from build123d import *

# Parameters (mm, degrees)
ESBO_O1_R                = 2.4
ESBO_O1_W                = 30
ESBO_O1_H                = 4
RESSALTO_EXTRUS_O1_DEPTH = 4
ESBO_O3_R                = 4
CORTE_EXTRUS_O1_DEPTH    = 6
FURO_COM_FOLGA_DE_M41_D  = 4.5
RESSALTO_EXTRUS_O2_DEPTH = 4
ESBO_O8_R                = 6
ESBO_O8_R_2              = 9
CORTE_EXTRUS_O4_DEPTH    = 5


with BuildPart() as part:
    # Esboço1 → Ressalto-extrusão1 (new body)
    with BuildSketch(Plane.XY):
        with BuildLine():
            Line((120, 130), (120, 140))
            ThreePointArc((120, 140), (122.928932188, 147.071067812), (130, 150))
            Line((130, 150), (50, 150))
            ThreePointArc((50, 150), (57.071067812, 147.071067812), (60, 140))
            Line((60, 140), (60, 130))
            Line((60, 130), (120, 130))
        make_face()
        with BuildLine():
            Line((0, 140), (0, 0))
            Line((0, 0), (400, 0))
            Line((400, 0), (400, 140))
            ThreePointArc((400, 140), (397.071067812, 147.071067812), (390, 150))
            Line((390, 150), (319, 150))
            Line((319, 150), (301, 150))
            Line((301, 150), (130, 150))
            ThreePointArc((130, 150), (122.928932188, 147.071067812), (120, 140))
            Line((120, 140), (120, 130))
            Line((120, 130), (60, 130))
            Line((60, 130), (60, 140))
            ThreePointArc((60, 140), (57.071067812, 147.071067812), (50, 150))
            Line((50, 150), (10, 150))
            ThreePointArc((10, 150), (2.928932188, 147.071067812), (0, 140))
        make_face()
        with Locations((30, 96.5)):
            Circle(ESBO_O1_R, mode=Mode.SUBTRACT)
        with Locations((30, 133.5)):
            Circle(ESBO_O1_R, mode=Mode.SUBTRACT)
        with Locations((100, 126)):
            Rectangle(ESBO_O1_W, ESBO_O1_H, mode=Mode.SUBTRACT)
        with BuildLine():
            ThreePointArc((365, 94.1), (362.6, 96.5), (365, 98.9))
            Line((365, 98.9), (375, 98.9))
            ThreePointArc((375, 98.9), (377.4, 96.5), (375, 94.1))
            Line((375, 94.1), (365, 94.1))
        make_face(mode=Mode.SUBTRACT)
        with Locations((200, 126)):
            Rectangle(ESBO_O1_W, ESBO_O1_H, mode=Mode.SUBTRACT)
        with Locations((300, 126)):
            Rectangle(ESBO_O1_W, ESBO_O1_H, mode=Mode.SUBTRACT)
        with BuildLine():
            ThreePointArc((365, 131.1), (362.6, 133.5), (365, 135.9))
            Line((365, 135.9), (375, 135.9))
            ThreePointArc((375, 135.9), (377.4, 133.5), (375, 131.1))
            Line((375, 131.1), (365, 131.1))
        make_face(mode=Mode.SUBTRACT)
    extrude(amount=RESSALTO_EXTRUS_O1_DEPTH)

    # Esboço3 → Corte-extrusão1 (cut)
    with BuildSketch(Plane.XY.offset(4)):
        with Locations((30, 115)):
            Circle(ESBO_O3_R)
        with BuildLine():
            Line((365, 119), (375, 119))
            ThreePointArc((375, 119), (379, 115), (375, 111))
            Line((375, 111), (365, 111))
            ThreePointArc((365, 111), (361, 115), (365, 119))
        make_face()
        with BuildLine():
            Line((40, 67.5), (60, 67.5))
            ThreePointArc((60, 67.5), (61.5, 66), (60, 64.5))
            Line((60, 64.5), (40, 64.5))
            ThreePointArc((40, 64.5), (38.5, 66), (40, 67.5))
        make_face()
        with BuildLine():
            Line((71, 36.5), (91, 36.5))
            ThreePointArc((91, 36.5), (92.5, 35), (91, 33.5))
            Line((91, 33.5), (71, 33.5))
            ThreePointArc((71, 33.5), (69.5, 35), (71, 36.5))
        make_face()
        with BuildLine():
            Line((71, 67.5), (91, 67.5))
            ThreePointArc((91, 67.5), (92.5, 66), (91, 64.5))
            Line((91, 64.5), (71, 64.5))
            ThreePointArc((71, 64.5), (69.5, 66), (71, 67.5))
        make_face()
        with BuildLine():
            Line((40, 36.5), (60, 36.5))
            ThreePointArc((60, 36.5), (61.5, 35), (60, 33.5))
            Line((60, 33.5), (40, 33.5))
            ThreePointArc((40, 33.5), (38.5, 35), (40, 36.5))
        make_face()
        with BuildLine():
            Line((55.5, 62), (75.5, 62))
            ThreePointArc((75.5, 62), (87, 50.5), (75.5, 39))
            Line((75.5, 39), (55.5, 39))
            ThreePointArc((55.5, 39), (44, 50.5), (55.5, 62))
        make_face()
    extrude(amount=-CORTE_EXTRUS_O1_DEPTH, mode=Mode.SUBTRACT)

    # Furo com folga de M41 (through all)
    with Locations(Plane(origin=(50, 12.5, 4), x_dir=(1, 0, 0), z_dir=(0, 0, 1))):
        with Locations((0, 0), (100, 0), (200, 0), (300, 0), (225, 62.5), (75, 62.5), (27, 127.5), (80, 127.5)):
            Hole(FURO_COM_FOLGA_DE_M41_D / 2)

    # Esboço5 → Ressalto-extrusão2 (add)
    with BuildSketch(Plane.XY.offset(4)):
        with BuildLine():
            Line((0, 140), (0, 148))
            ThreePointArc((0, 148), (2.928932188, 155.071067812), (10, 158))
            Line((10, 158), (390, 158))
            ThreePointArc((390, 158), (397.071067812, 155.071067812), (400, 148))
            Line((400, 148), (400, 140))
            ThreePointArc((400, 140), (397.071067812, 147.071067812), (390, 150))
            Line((390, 150), (10, 150))
            ThreePointArc((10, 150), (2.928932188, 147.071067812), (0, 140))
        make_face()
    extrude(amount=-RESSALTO_EXTRUS_O2_DEPTH)

    # Esboço8 → Corte-extrusão4 (cut, through all)
    with BuildSketch(Plane.XY):
        with Locations((150, 144)):
            Circle(ESBO_O8_R)
        with Locations((310, 144)):
            Circle(ESBO_O8_R_2)
    extrude(amount=CORTE_EXTRUS_O4_DEPTH, mode=Mode.SUBTRACT)


solid = part.part
Source: CAD feature listing. Evaluate the final solid. Frame: model axes, mm. A direction names the side the tool comes from. Round coordinates to 2 decimals unless told otherwise and drop trailing zeros. Order: outer loops, then holes, each group sorted by start corner. A loop starts at its lowest first (then second) coordinate and runs counter-clockwise, first axis right, second up. Notation, with made-up numbers: (87.5, -3) -> (119.5, -3) arc R21 ccw to (119.5, 27) -> close; hole circle Ø10 at (59, 69.5). An arc over 180 degrees is marked (long way). Answer as CSV lines item,"result".
Item 1: Section C-C, the plane z = 2.4. Count the separate pieces of the cut face and the enclosed holes in it, plus the area to 3 significant figures.
A:
separate pieces,"1"
enclosed holes,"24"
area,"60,800 mm²"
Item 2: Section B-B, the plane x = 307. Return loops of the section in (y, z).
A:
outline,"(0, 0) -> (124, 0) -> (124, 4) -> (0, 4) -> close; (128, 0) -> (135.51, 0) -> (135.51, 4) -> (128, 4) -> close; (152.49, 0) -> (158, 0) -> (158, 4) -> (152.49, 4) -> close"
Item 3: Pin query (flat end, axial travel): pin 1 Ø2.5 at (x, y) = (130, 140) entering from -Z; pin 2 Ø2 at (x, z) = (372.5, 1.5) entering from -Y. Return the tip coordinate at first contact, or that it passes through.
A:
pin 1,"through"
pin 2,"y = 0"
Item 4: Line query: L1, parallel to Y at x = 310, z = 1.95; L2, parallel to Y at x = 30, z = 2.45; L3, parallel to X at y = 12, z = 1.7. Output: solid intervals per line, ascending.
A:
L1,"0 to 124, 128 to 135, 153 to 158"
L2,"0 to 94.1, 98.9 to 111, 119 to 131.1, 135.9 to 158"
L3,"0 to 47.81, 52.19 to 147.81, 152.19 to 247.81, 252.19 to 347.81, 352.19 to 400"
Item 5: Pull-direction query (Y, two-part tool) for faces 3 (the face through (203, 80, 0)), 4 (the face through (396.99, 155.15, 2.03)), 5 (the face through (29.479, 118.966, 2.028)); classes: pulls with the +Y half, pulls with the -Y half, needs draft (parallel to the pull), parting line crosses it, or undercut.
A:
face 3,"needs draft"
face 4,"pulls with the +Y half"
face 5,"undercut"
Item 6: Section A-A, the plane x = 200. Return loops of the section in (y, z).
A:
outline,"(0, 0) -> (124, 0) -> (124, 4) -> (0, 4) -> close; (128, 0) -> (158, 0) -> (158, 4) -> (128, 4) -> close"
Item 7: Reachability of faces 1 (the face through (203, 80, 4)), 2 (the face through (86.997, 50.753, 2.028)) from +Z, -Z, +X, -X, +Y, -Y: full face, straight path, thin tool, end or side. Return the list, or none.
A:
face 1,"+Z, +X, -X, +Y, -Y"
face 2,"+Z, -Z"
